from build123d import *

# Parameters (mm, degrees)
SKETCH_1_W          = 44.8
SKETCH_1_H          = 41.2
EXTRUDE_1_DEPTH     = 4.6
SKETCH_3_W          = 41.6
SKETCH_3_H          = 38
CUT_EXTRUDE_1_DEPTH = 3
SKETCH_4_W          = 10.6
SKETCH_4_H          = 7.6
CUT_EXTRUDE_2_DEPTH = 5.6
FILLET_1_R          = 2.6
FILLET_2_R          = 1
SKETCH_5_R          = 15
EXTRUDE_2_DEPTH     = 2.6


with BuildPart() as part:
    # ｽｹｯﾁ1 → ﾎﾞｽ - 押し出し1 (new body)
    with BuildSketch(Plane(origin=(0, 0, 0), x_dir=(1, 0, 0), z_dir=(0, 1, 0))):
        Rectangle(SKETCH_1_W, SKETCH_1_H)
    extrude(amount=EXTRUDE_1_DEPTH)

    # ｽｹｯﾁ3 → ｶｯﾄ - 押し出し1 (cut)
    with BuildSketch(Plane(origin=(0, 0, 0), x_dir=(-1, 0, 0), z_dir=(0, -1, 0))):
        Rectangle(SKETCH_3_W, SKETCH_3_H)
    extrude(amount=-CUT_EXTRUDE_1_DEPTH, mode=Mode.SUBTRACT)

    # ｽｹｯﾁ4 → ｶｯﾄ - 押し出し2 (cut, through all)
    with BuildSketch(Plane(origin=(0, 4.6, 0), x_dir=(1, 0, 0), z_dir=(0, 1, 0))):
        with Locations((17.1, -16.8)):
            Rectangle(SKETCH_4_W, SKETCH_4_H)
        with Locations((17.1, 16.8)):
            Rectangle(SKETCH_4_W, SKETCH_4_H)
        with Locations((-17.1, -16.8)):
            Rectangle(SKETCH_4_W, SKETCH_4_H)
        with Locations((-17.1, 16.8)):
            Rectangle(SKETCH_4_W, SKETCH_4_H)
    extrude(amount=-CUT_EXTRUDE_2_DEPTH, mode=Mode.SUBTRACT)

    # ﾌｨﾚｯﾄ1
    fillet_1_edges = [part.edges().sort_by_distance(p)[0] for p in [
        (22.4, 4.6, 0),
        (0, 4.6, -20.6),
        (0, 4.6, 20.6),
        (-22.4, 4.6, 0),
    ]]
    fillet(fillet_1_edges, radius=FILLET_1_R)

    # ﾌｨﾚｯﾄ2
    fillet_2_edges = [part.edges().sort_by_distance(p)[0] for p in [
        (0, 3, 19),
        (20.8, 3, 0),
        (-20.8, 3, 0),
        (0, 3, -19),
    ]]
    fillet(fillet_2_edges, radius=FILLET_2_R)

    # ｽｹｯﾁ5 → ﾎﾞｽ - 押し出し2 (add)
    with BuildSketch(Plane(origin=(0, 4.6, 0), x_dir=(1, 0, 0), z_dir=(0, 1, 0))):
        Circle(SKETCH_5_R)
    extrude(amount=EXTRUDE_2_DEPTH)


solid = part.part
Geometry check sheet. Reference: the model listing, model coordinates, mm. A direction names the side the tool comes from. Coordinates: 2 decimals unless noted, no trailing zeros. Order: outer loops, then holes, each group sorted by start corner. A loop starts at its lowest first (then second) coordinate and runs counter-clockwise, first axis right, second up. Notation, with made-up numbers: M 6,61.5 L 51,61.5 A32 cw 51,94.5 Z; hole C 89.25,-31 d2. An arc over 180 degrees is marked long. Use CSV: the item, a comma, the result in double quotes.
Item 1: Cross-section at B-B on z = -12. Record the cut outline in (x, y), then the cut area to 3 significant figures.
Returned:
outline,"M -22.4,0 L -20.8,0 L -20.8,2 A1 cw -19.8,3 L 19.8,3 A1 cw 20.8,2 L 20.8,0 L 22.4,0 L 22.4,2 A2.6 ccw 19.8,4.6 L 9,4.6 L 9,7.2 L -9,7.2 L -9,4.6 L -19.8,4.6 A2.6 ccw -22.4,2 Z"
area,"126 mm2"
Item 2: Cross-section at D-D on y = 4. Record the cut outline in (x, z), then the cut area to 3 significant figures.
Returned:
outline,"M -21.46,-13 L -11.8,-13 L -11.8,-19.66 L 11.8,-19.66 L 11.8,-13 L 21.46,-13 L 21.46,13 L 11.8,13 L 11.8,19.66 L -11.8,19.66 L -11.8,13 L -21.46,13 Z"
area,"1,430 mm2"
Item 3: Cross-section at C-C on x = 0. Record the cut outline in (y, z).
Returned:
outline,"M 0,-20.6 L 2,-20.6 A2.6 ccw 4.6,-18 L 4.6,-15 L 7.2,-15 L 7.2,15 L 4.6,15 L 4.6,18 A2.6 ccw 2,20.6 L 0,20.6 L 0,19 L 2,19 A1 cw 3,18 L 3,-18 A1 cw 2,-19 L 0,-19 Z"
Item 4: Gauge pin test, flat ends, axial feed: pin 1 Ø4 at (x, y) = (5, 2.5) entering from -Z; pin 2 Ø2 at (y, z) = (4.5, 3) entering from -X; pin 3 Ø3 at (y, z) = (4.5, 4.5) entering from +X; pin 4 Ø3.5 at (y, z) = (3, 18.5) entering from -X. Record the tip position at first contact, or that the pin passes through.
Returned:
pin 1,"stops at z = -20.6"
pin 2,"stops at x = -21.92"
pin 3,"stops at x = 22.2"
pin 4,"stops at x = -11.8"
Item 5: Thickness scan on line 1 along X through (y, z) = (1.25, -11.5); line 2 along Y through (x, z) = (1, -10.5); line 3 along Y through (x, z) = (-3.5, 16.5). Record the ranges inside material, lowest first.
Returned:
line 1,"x = -22.4 to -20.8, 20.8 to 22.4"
line 2,"y = 3 to 7.2"
line 3,"y = 3 to 4.6"
Item 6: Tool access check on faces 1 (the flat face through (11.8, 3.4, 17.7)), 2 (the flat face through (-11.8, 3.4, 17.7)), 3 (the flat face through (18.2, 3.4, -13)), 4 (the flat face through (-18.4, 3.4, -13)), 5 (the cylindrical face through (-0.165, 2.715, 18.699)). Record the directions out of +Z, -Z, +X, -X, +Y, -Y that give a thin tool (end or side, any length) a straight path to the whole face; none if there is none.
Returned:
face 1,"+Z, +X, +Y, -Y"
face 2,"+Z, -X, +Y, -Y"
face 3,"-Z, +X, +Y, -Y"
face 4,"-Z, -X, +Y, -Y"
face 5,"+X, -X, -Y"
Item 7: Mould release check, pull along X, two halves, no side actions. Record for faces 6 (the cylindrical face through (-0.165, 2.715, -18.699)), 7 (the cylindrical face through (-20.499, 2.715, -0.182)), 8 (the flat face through (11.8, 3.4, -17.6)), 9 (the flat face through (-22.4, 1, 0)): pulls with the +X half, pulls with the -X half, needs draft (parallel to the pull), parting line crosses it, or undercut.
Returned:
face 6,"needs draft"
face 7,"undercut"
face 8,"pulls with the +X half"
face 9,"pulls with the -X half"
Item 8: Cross-section at A-A on y = 0.5. Record the cut outline in (x, z), then the cut area to 3 significant figures.
Returned:
outline,"M -22.4,-13 L -20.8,-13 L -20.8,13 L -22.4,13 Z; M -11.8,-20.6 L 11.8,-20.6 L 11.8,-19 L -11.8,-19 Z; M -11.8,19 L 11.8,19 L 11.8,20.6 L -11.8,20.6 Z; M 20.8,-13 L 22.4,-13 L 22.4,13 L 20.8,13 Z"
area,"159 mm2"
